Geometry: final body of the model. Coordinates: model frame, mm. A direction names the side the tool comes from. Coordinates: 2 decimals unless noted, no trailing zeros. Write each loop counter-clockwise with the first axis right and the second up, starting at its lowest first coordinate (ties: lowest second). Pieces come first, ordered by that corner, then holes.
from build123d import *

# Parameters (mm, degrees)
SKETCH2_W                   = 60
SKETCH2_H                   = 80
BOSS_EXTRUDE2_DEPTH         = 16
SKETCH6_W                   = 52
SKETCH6_H                   = 72
CUT_EXTRUDE1_DEPTH          = 12
CUT_EXTRUDE2_DEPTH          = 16
CUT_EXTRUDE2_DEPTH_BACK     = 106
SKETCH7_W                   = 22
SKETCH7_H                   = 8
SKETCH8_W                   = 4
SKETCH8_H                   = 10
BOSS_EXTRUDE3_DEPTH         = 12
FILLET1_RADIUS              = 5
FILLET1_LENGTH              = 4
FILLET2_RADIUS              = 5
FILLET2_LENGTH              = 4
FILLET3_RADIUS              = 5
FILLET3_LENGTH              = 4
FILLET4_RADIUS              = 5
FILLET4_LENGTH              = 4
BOSS_EXTRUDE4_START         = -2
SKETCH9_R                   = 2.5
BOSS_EXTRUDE4_DEPTH         = 26
MIRROR2_START               = -2
MIRROR2_COPY_1_SKETCH_R     = 2.5
MIRROR2_COPY_1_DEPTH        = 26
FILLET1_OF_MIRROR2_2_RADIUS = 5
FILLET1_OF_MIRROR2_2_LENGTH = 4
FILLET2_OF_MIRROR2_2_RADIUS = 5
FILLET2_OF_MIRROR2_2_LENGTH = 4
FILLET3_OF_MIRROR2_2_RADIUS = 5
FILLET3_OF_MIRROR2_2_LENGTH = 4
FILLET4_OF_MIRROR2_2_RADIUS = 5
FILLET4_OF_MIRROR2_2_LENGTH = 4


with BuildPart() as part:
    # Sketch2 → Boss-Extrude2 (new body)
    with BuildSketch(Plane(origin=(0, 0, 0), x_dir=(1, 0, 0), z_dir=(0, 1, 0))):
        Rectangle(SKETCH2_W, SKETCH2_H)
    extrude(amount=BOSS_EXTRUDE2_DEPTH)

    # Sketch6 → Cut-Extrude1 (cut)
    with BuildSketch(Plane(origin=(0, 16, 0), x_dir=(1, 0, 0), z_dir=(0, 1, 0))):
        Rectangle(SKETCH6_W, SKETCH6_H)
    extrude(amount=-CUT_EXTRUDE1_DEPTH, mode=Mode.SUBTRACT)

    # Sketch7 → Cut-Extrude2 (cut, two sides: drawn at the far end of the back side and taken through both)
    with BuildSketch(Plane(origin=(0, 0, -40), x_dir=(-1, 0, 0), z_dir=(0, 0, -1)).offset(-CUT_EXTRUDE2_DEPTH_BACK)):
        with Locations((-14, 8)):
            Rectangle(SKETCH7_W, SKETCH7_H)
        with Locations((14, 8)):
            Rectangle(SKETCH7_W, SKETCH7_H)
    extrude(amount=CUT_EXTRUDE2_DEPTH + CUT_EXTRUDE2_DEPTH_BACK, mode=Mode.SUBTRACT)

    # Sketch8 → Boss-Extrude3 (add)
    with BuildSketch(Plane(origin=(30, 0, 0), x_dir=(0, 0, -1), z_dir=(1, 0, 0))):
        with Locations((-33, 8.303078398)):
            Rectangle(SKETCH8_W, SKETCH8_H)
        with Locations((-7, 8.355173675)):
            Rectangle(SKETCH8_W, SKETCH8_H)
        with Locations((7, 8.355173675)):
            Rectangle(SKETCH8_W, SKETCH8_H)
        with Locations((33, 8.303078398)):
            Rectangle(SKETCH8_W, SKETCH8_H)
    boss_extrude3 = extrude(amount=BOSS_EXTRUDE3_DEPTH)

    # Fillet1: full round fillet: the end face becomes a half cylinder, R = half its width
    fillet1_face = Plane((42, 8.303078398, 33), x_dir=(0, 0, 1), z_dir=(1, 0, 0))  # on the end face: x along it, z out of the body
    fillet1_slab = fillet1_face.offset(-FILLET1_RADIUS / 2) * Box(FILLET1_LENGTH, 2 * FILLET1_RADIUS, FILLET1_RADIUS, mode=Mode.PRIVATE)  # the body's end, R deep
    fillet1_round = Plane((37, 8.303078398, 33), x_dir=(1, 0, 0), z_dir=(0, 0, 1)) * Cylinder(FILLET1_RADIUS, FILLET1_LENGTH, mode=Mode.PRIVATE)  # its axis R under the face
    add(fillet1_slab - fillet1_round, mode=Mode.SUBTRACT)

    # Fillet2: full round fillet: the end face becomes a half cylinder, R = half its width
    fillet2_face = Plane((42, 8.355173675, 7), x_dir=(0, 0, 1), z_dir=(1, 0, 0))  # on the end face: x along it, z out of the body
    fillet2_slab = fillet2_face.offset(-FILLET2_RADIUS / 2) * Box(FILLET2_LENGTH, 2 * FILLET2_RADIUS, FILLET2_RADIUS, mode=Mode.PRIVATE)  # the body's end, R deep
    fillet2_round = Plane((37, 8.355173675, 7), x_dir=(1, 0, 0), z_dir=(0, 0, 1)) * Cylinder(FILLET2_RADIUS, FILLET2_LENGTH, mode=Mode.PRIVATE)  # its axis R under the face
    add(fillet2_slab - fillet2_round, mode=Mode.SUBTRACT)

    # Fillet3: full round fillet: the end face becomes a half cylinder, R = half its width
    fillet3_face = Plane((42, 8.355173675, -7), x_dir=(0, 0, -1), z_dir=(1, 0, 0))  # on the end face: x along it, z out of the body
    fillet3_slab = fillet3_face.offset(-FILLET3_RADIUS / 2) * Box(FILLET3_LENGTH, 2 * FILLET3_RADIUS, FILLET3_RADIUS, mode=Mode.PRIVATE)  # the body's end, R deep
    fillet3_round = Plane((37, 8.355173675, -7), x_dir=(1, 0, 0), z_dir=(0, 0, -1)) * Cylinder(FILLET3_RADIUS, FILLET3_LENGTH, mode=Mode.PRIVATE)  # its axis R under the face
    add(fillet3_slab - fillet3_round, mode=Mode.SUBTRACT)

    # Fillet4: full round fillet: the end face becomes a half cylinder, R = half its width
    fillet4_face = Plane((42, 8.303078398, -33), x_dir=(0, 0, -1), z_dir=(1, 0, 0))  # on the end face: x along it, z out of the body
    fillet4_slab = fillet4_face.offset(-FILLET4_RADIUS / 2) * Box(FILLET4_LENGTH, 2 * FILLET4_RADIUS, FILLET4_RADIUS, mode=Mode.PRIVATE)  # the body's end, R deep
    fillet4_round = Plane((37, 8.303078398, -33), x_dir=(1, 0, 0), z_dir=(0, 0, -1)) * Cylinder(FILLET4_RADIUS, FILLET4_LENGTH, mode=Mode.PRIVATE)  # its axis R under the face
    add(fillet4_slab - fillet4_round, mode=Mode.SUBTRACT)

    # Sketch9 → Boss-Extrude4 (add)
    with BuildSketch(Plane(origin=(0, 0, 31), x_dir=(-1, 0, 0), z_dir=(0, 0, -1)).offset(BOSS_EXTRUDE4_START)):
        with Locations(Location((-37, 8.303078398, 0), (0, 0, 180))):
            Circle(SKETCH9_R)
    boss_extrude4 = extrude(amount=BOSS_EXTRUDE4_DEPTH)

    # Mirror1: Boss-Extrude4 across plane
    add(boss_extrude4.mirror(Plane(origin=(0, 0, 0), x_dir=(1, 0, 0), z_dir=(0, 0, -1))))

    # Mirror2: Boss-Extrude3, Boss-Extrude4 across plane
    add(boss_extrude3.mirror(Plane(origin=(0, 0, 0), x_dir=(0, 0, 1), z_dir=(1, 0, 0))))
    add(boss_extrude4.mirror(Plane(origin=(0, 0, 0), x_dir=(0, 0, 1), z_dir=(1, 0, 0))))

    # Mirror2 copy 1 sketch → Mirror2 copy 1 (add)
    with BuildSketch(Plane.XY.offset(-31).offset(MIRROR2_START)):
        with Locations(Location((-37, 8.303078398, 0), (0, 0, 180))):
            Circle(MIRROR2_COPY_1_SKETCH_R)
    extrude(amount=MIRROR2_COPY_1_DEPTH)

    # Fillet1 of Mirror2 2: full round fillet: the end face becomes a half cylinder, R = half its width
    fillet1_of_mirror2_2_face = Plane((-42, 8.303078398, 33), x_dir=(0, 0, 1), z_dir=(-1, 0, 0))  # on the end face: x along it, z out of the body
    fillet1_of_mirror2_2_slab = fillet1_of_mirror2_2_face.offset(-FILLET1_OF_MIRROR2_2_RADIUS / 2) * Box(FILLET1_OF_MIRROR2_2_LENGTH, 2 * FILLET1_OF_MIRROR2_2_RADIUS, FILLET1_OF_MIRROR2_2_RADIUS, mode=Mode.PRIVATE)  # the body's end, R deep
    fillet1_of_mirror2_2_round = Plane((-37, 8.303078398, 33), x_dir=(-1, 0, 0), z_dir=(0, 0, 1)) * Cylinder(FILLET1_OF_MIRROR2_2_RADIUS, FILLET1_OF_MIRROR2_2_LENGTH, mode=Mode.PRIVATE)  # its axis R under the face
    add(fillet1_of_mirror2_2_slab - fillet1_of_mirror2_2_round, mode=Mode.SUBTRACT)

    # Fillet2 of Mirror2 2: full round fillet: the end face becomes a half cylinder, R = half its width
    fillet2_of_mirror2_2_face = Plane((-42, 8.355173675, 7), x_dir=(0, 0, 1), z_dir=(-1, 0, 0))  # on the end face: x along it, z out of the body
    fillet2_of_mirror2_2_slab = fillet2_of_mirror2_2_face.offset(-FILLET2_OF_MIRROR2_2_RADIUS / 2) * Box(FILLET2_OF_MIRROR2_2_LENGTH, 2 * FILLET2_OF_MIRROR2_2_RADIUS, FILLET2_OF_MIRROR2_2_RADIUS, mode=Mode.PRIVATE)  # the body's end, R deep
    fillet2_of_mirror2_2_round = Plane((-37, 8.355173675, 7), x_dir=(-1, 0, 0), z_dir=(0, 0, 1)) * Cylinder(FILLET2_OF_MIRROR2_2_RADIUS, FILLET2_OF_MIRROR2_2_LENGTH, mode=Mode.PRIVATE)  # its axis R under the face
    add(fillet2_of_mirror2_2_slab - fillet2_of_mirror2_2_round, mode=Mode.SUBTRACT)

    # Fillet3 of Mirror2 2: full round fillet: the end face becomes a half cylinder, R = half its width
    fillet3_of_mirror2_2_face = Plane((-42, 8.355173675, -7), x_dir=(0, 0, -1), z_dir=(-1, 0, 0))  # on the end face: x along it, z out of the body
    fillet3_of_mirror2_2_slab = fillet3_of_mirror2_2_face.offset(-FILLET3_OF_MIRROR2_2_RADIUS / 2) * Box(FILLET3_OF_MIRROR2_2_LENGTH, 2 * FILLET3_OF_MIRROR2_2_RADIUS, FILLET3_OF_MIRROR2_2_RADIUS, mode=Mode.PRIVATE)  # the body's end, R deep
    fillet3_of_mirror2_2_round = Plane((-37, 8.355173675, -7), x_dir=(-1, 0, 0), z_dir=(0, 0, -1)) * Cylinder(FILLET3_OF_MIRROR2_2_RADIUS, FILLET3_OF_MIRROR2_2_LENGTH, mode=Mode.PRIVATE)  # its axis R under the face
    add(fillet3_of_mirror2_2_slab - fillet3_of_mirror2_2_round, mode=Mode.SUBTRACT)

    # Fillet4 of Mirror2 2: full round fillet: the end face becomes a half cylinder, R = half its width
    fillet4_of_mirror2_2_face = Plane((-42, 8.303078398, -33), x_dir=(0, 0, -1), z_dir=(-1, 0, 0))  # on the end face: x along it, z out of the body
    fillet4_of_mirror2_2_slab = fillet4_of_mirror2_2_face.offset(-FILLET4_OF_MIRROR2_2_RADIUS / 2) * Box(FILLET4_OF_MIRROR2_2_LENGTH, 2 * FILLET4_OF_MIRROR2_2_RADIUS, FILLET4_OF_MIRROR2_2_RADIUS, mode=Mode.PRIVATE)  # the body's end, R deep
    fillet4_of_mirror2_2_round = Plane((-37, 8.303078398, -33), x_dir=(-1, 0, 0), z_dir=(0, 0, -1)) * Cylinder(FILLET4_OF_MIRROR2_2_RADIUS, FILLET4_OF_MIRROR2_2_LENGTH, mode=Mode.PRIVATE)  # its axis R under the face
    add(fillet4_of_mirror2_2_slab - fillet4_of_mirror2_2_round, mode=Mode.SUBTRACT)


solid = part.part
Item 1: Section D-D, the plane z = -13. Output: boundary loops of the cut face in (x, y).
Derived:
outline: circle Ø5 at (-37, 8.3); (-30, 0) - (30, 0) - (30, 16) - (26, 16) - (26, 4) - (-26, 4) - (-26, 16) - (-30, 16) - close; circle Ø5 at (37, 8.3)
Item 2: Section B-B, the plane y = 14.75. Output: boundary loops of the cut face in (x, z).
Derived:
outline: (-30, -40) - (30, -40) - (30, 40) - (-30, 40) - close; hole (-26, -36) - (26, -36) - (26, 36) - (-26, 36) - close
Item 3: Material intervals for probe 1 along X at (y, z) = (8.5, 17); probe 2 along Z at (x, y) = (33, 6.25); probe 3 along Z at (x, y) = (-5, 14.75), sorted ascending.
Derived:
probe 1: x = -39.49 to -34.51, -30 to -26, 26 to 30, 34.51 to 39.49
probe 2: z = -35 to -31, -9 to -5, 5 to 9, 31 to 35
probe 3: z = -40 to -36, 36 to 40
Item 4: Set-up query: faces 3 (the flat face through (36, 8, 5)), 4 (the flat face through (-34.6, 7.1, 31)), 5 (the flat face through (33, 13.355, -7)), 6 (the flat face through (-33, 13.355, 7)). Return all of +Z, -Z, +X, -X, +Y, -Y with unobstructed straight access to the full face (end or side cutting, diameter ignored); none if empty.
Derived:
face 3: +X, +Y, -Y
face 4: none
face 5: +Z, -Z, +X, +Y
face 6: +Z, -Z, -X, +Y
Item 5: Pull-direction query (Z, two-part tool) for faces 1 (the flat face through (34.58, 9.4, -9)), 2 (the cylindrical face through (-42, 8.4, 33)); classes: released by +Z, released by -Z, zero draft, split by the parting line, or undercut.
Derived:
face 1: undercut
face 2: zero draft
Item 6: Pin query (flat end, axial travel): pin 1 (5 mm diameter, centred on x = 37.5, y = 6.5, fed in from +Z); pin 2 (3 mm diameter, centred on y = 8.5, z = -38.5, fed in from +X); pin 3 (1.2 mm diameter, centred on x = 35, z = 6.5, fed in from +Y). Return the tip coordinate at first contact, or that it passes through.
Derived:
pin 1: stops at z = 35
pin 2: stops at x = 30
pin 3: stops at y = 13.36
Item 7: Section C-C, the plane z = -32.5. Output: boundary loops of the cut face in (x, y), plus the area to 3 significant figures.
Derived:
outline: (-37, 3.3) - (-30, 3.3) - (-30, 0) - (30, 0) - (30, 3.3) - (37, 3.3) arc R5 ccw to (37, 13.3) - (30, 13.3) - (30, 16) - (26, 16) - (26, 4) - (-26, 4) - (-26, 16) - (-30, 16) - (-30, 13.3) - (-37, 13.3) arc R5 ccw to start
area: 555 mm2
Item 8: Section A-A, the plane x = 5.5. Output: boundary loops of the cut face in (y, z).
Derived:
outline: (0, -40) - (4, -40) - (4, 40) - (0, 40) - close; (12, -40) - (16, -40) - (16, -36) - (12, -36) - close; (12, 36) - (16, 36) - (16, 40) - (12, 40) - close
